Check sheet for the modelled part. Datum: model origin and axes. Units: mm. Face numbers are marked on the shaded views. A direction names the side the tool comes from. Give positions to 0.01 mm unless a question says otherwise; leave off trailing zeros. Order: outer loops, then holes, each group sorted by start corner. A loop starts at its lowest first (then second) coordinate and runs counter-clockwise, first axis right, second up. Notation, with made-up numbers: (14, 83.5) -> (21, 83.5) arc R12 ccw to (21, 100.5) -> close; hole circle Ø5 at (87.25, 36.25). An arc over 180 degrees is marked (long way). Answer in a Markdown table with one row per item. Add a question column.
(1) Release check for a two-part mould opening along Z. For the marked faces 1, 2 and 3 record: released by +Z, released by -Z, zero draft, split by the parting line, or undercut.
(2) Cross-section at D-D (y = -4). Record the cut outline in (x, z) (1 decimal).
(3) Cross-section at A-A (y = 0). Record the cut outline in (x, z) (1 decimal), then the cut area to 3 significant figures.
(4) Thickness scan on L1, parallel to Z at x = 2.5, y = 3.75 (1 decimal); L2, parallel to Y at x = 0, z = 5; L3, parallel to Y at x = 0, z = 8.75. Record the ranges inside material, lowest first. Write a range as [from, to].
(5) Set-up check for the marked faces 4 and 5: record each of +Z, -Z, +X, -X, +Y, -Y from which the full face is reachable in a straight line by a thin tool's end or side.
(6) Cross-section at C-C (z = 4). Record the cut outline in (x, y).
(7) Go/stop test with a flat-tipped pin: pin 1 (2 mm diameter, centred on x = -3, z = 3, fed in from +Y). Record where the tip stops, or that it passes through.
```python
from build123d import *

# Parameters (mm, degrees)
SKETCH1_R           = 3.81
SKETCH1_R_2         = 3.2385
BOSS_EXTRUDE1_DEPTH = 10.795
SKETCH3_R           = 5.08
SKETCH3_R_2         = 3.81
BOSS_EXTRUDE2_DEPTH = 1.8415
SKETCH4_R           = 5.08
SKETCH4_R_2         = 3.81
BOSS_EXTRUDE3_DEPTH = 4.3815


with BuildPart() as part:
    # Sketch1 → Boss-Extrude1 (new body)
    with BuildSketch(Plane.XY):
        Circle(SKETCH1_R)
        Circle(SKETCH1_R_2, mode=Mode.SUBTRACT)
    extrude(amount=BOSS_EXTRUDE1_DEPTH)

    # Sketch3 → Boss-Extrude2 (add)
    with BuildSketch(Plane.XY.offset(1.8415)):
        Circle(SKETCH3_R)
        Circle(SKETCH3_R_2, mode=Mode.SUBTRACT)
    extrude(amount=-BOSS_EXTRUDE2_DEPTH)

    # Sketch4 → Boss-Extrude3 (add)
    with BuildSketch(Plane.XY.offset(6.4135)):
        Circle(SKETCH4_R)
        Circle(SKETCH4_R_2, mode=Mode.SUBTRACT)
    extrude(amount=BOSS_EXTRUDE3_DEPTH)


solid = part.part
```
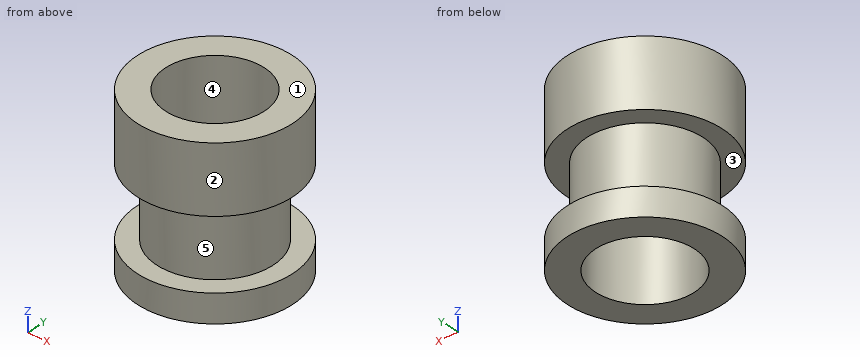
Answer below:
| question | item | result |
|---|---|---|
| 1 | face 1 | released by +Z |
| 1 | face 2 | zero draft |
| 1 | face 3 | undercut |
| 2 | outline | (-3.1, 0) -> (3.1, 0) -> (3.1, 1.8) -> (-3.1, 1.8) -> close; (-3.1, 6.4) -> (3.1, 6.4) -> (3.1, 10.8) -> (-3.1, 10.8) -> close |
| 3 | outline | (-5.1, 0) -> (-3.2, 0) -> (-3.2, 10.8) -> (-5.1, 10.8) -> (-5.1, 6.4) -> (-3.8, 6.4) -> (-3.8, 1.8) -> (-5.1, 1.8) -> close; (3.2, 0) -> (5.1, 0) -> (5.1, 1.8) -> (3.8, 1.8) -> (3.8, 6.4) -> (5.1, 6.4) -> (5.1, 10.8) -> (3.2, 10.8) -> close |
| 3 | area | 28.1 mm² |
| 4 | L1 | z = [0, 1.8], [6.4, 10.8] |
| 4 | L2 | y = [-3.81, -3.24], [3.24, 3.81] |
| 4 | L3 | y = [-5.08, -3.24], [3.24, 5.08] |
| 5 | face 4 | +Z, -Z |
| 5 | face 5 | none |
| 6 | outline | circle Ø7.62 at (0, 0); hole circle Ø6.48 at (0, 0) |
| 7 | pin 1 | stops at y = 3.24 |
